For this review, use the dimensioned drawing (mm, ordinates from the lowest corner) and the shaded views. A direction names the side the tool comes from. Give positions to 0.01 mm unless a question says otherwise; leave off trailing zeros. Loops run counter-clockwise (first coordinate to the right, second up) from the corner with the lowest first, then second, coordinate; pieces in that order, holes last. Notation, with made-up numbers: M 55.5,89 L 114.5,89 A21 cw 114.5,112 Z; hole C -33.5,11 d9. An arc over 180 degrees is marked long. Use CSV: the item, a comma, the result in double quotes. Start each with the question number.
1. Insertion check: P1, Ø2, axis at y = 1.5, z = 8, coming from the +X side; P2, Ø5, axis at y = 4.5, z = 14, coming from the -X side; P3, Ø6, axis at x = 9.5, z = 13, coming from the -Y side. Each pin has a flat end and moves straight along its axis. Give the tip position at first contact, or say it passes through.
2. Take a section at A-A, the plane y = 9. Write out the cut boundary in (x, z), and give its area (3 significant figures).
3. The part is to be moulded in two halves that separate along X. For the marked faces 3, 4 and 5, say which applies: pulls with the +X half, pulls with the -X half, needs draft (parallel to the pull), parting line crosses it, or undercut.
4. Take a section at C-C, the plane z = 10. Write out the cut boundary in (x, y) (3 decimals), and give its area (3 significant figures).
5. Take a section at D-D, the plane y = 6.75. Write out the cut boundary in (x, z).
6. Tool access review of the marked faces 1 and 2: name each direction out of +Z, -Z, +X, -X, +Y, -Y from which nothing blocks a thin tool from reaching the whole face with its end or side.
7. To check wall thickness, follow line 1 (X direction, y = 3, z = 10); line 2 (X direction, y = 9.75, z = 10); line 3 (Z direction, x = 9.25, y = 3.75). State the ranges of each line that lie inside material, in increasing order. Write a range as [from, to].
8. Take a section at B-B, the plane x = 10. Write out the cut boundary in (y, z) (3 decimals), and give its area (3 significant figures).
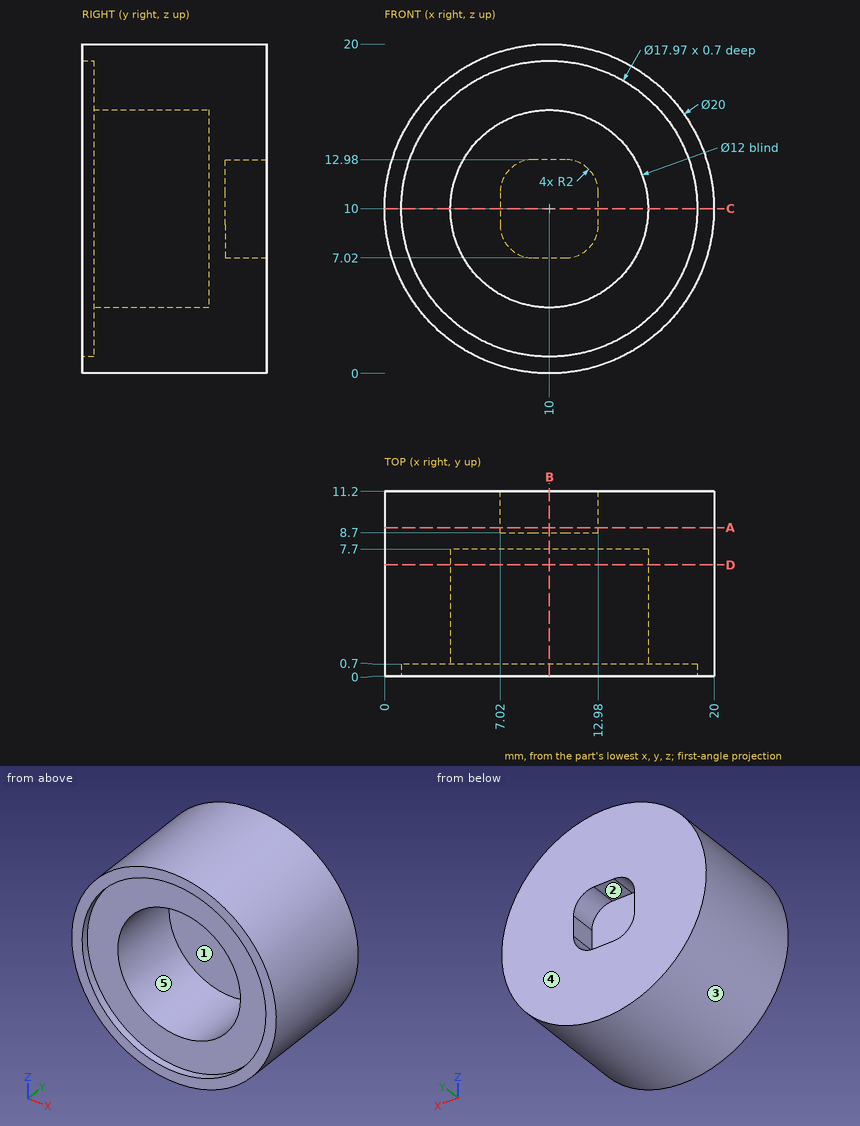
Result set:
1,P1,"x = 19.95"
1,P2,"x = 0.11"
1,P3,"y = 0.7"
2,outline,"C 10,10 d20; hole M 7.02,9.02 A2 ccw 9.02,7.02 L 10.98,7.02 A2 ccw 12.98,9.02 L 12.98,10.98 A2 ccw 10.98,12.98 L 9.02,12.98 A2 ccw 7.02,10.98 Z"
2,area,"282 mm2"
3,face 3,"parting line crosses it"
3,face 4,"needs draft"
3,face 5,"undercut"
4,outline,"M 0,0 L 1.015,0 L 1.015,0.7 L 4,0.7 L 4,7.7 L 16,7.7 L 16,0.7 L 18.985,0.7 L 18.985,0 L 20,0 L 20,11.2 L 12.98,11.2 L 12.98,8.7 L 7.02,8.7 L 7.02,11.2 L 0,11.2 Z"
4,area,"113 mm2"
5,outline,"C 10,10 d20; hole C 10,10 d12"
6,face 1,"-Y"
6,face 2,"+Y"
7,line 1,"[0, 4], [16, 20]"
7,line 2,"[0, 7.02], [12.98, 20]"
7,line 3,"[0.03, 4.05], [15.95, 19.97]"
8,outline,"M 0,0 L 11.2,0 L 11.2,7.02 L 8.7,7.02 L 8.7,12.98 L 11.2,12.98 L 11.2,20 L 0,20 L 0,18.985 L 0.7,18.985 L 0.7,16 L 7.7,16 L 7.7,4 L 0.7,4 L 0.7,1.015 L 0,1.015 Z"
8,area,"113 mm2"
